Design review of the part built by this model. Coordinates are the model's own, in mm. Coordinates: 2 decimals unless noted, no trailing zeros. Loops run counter-clockwise (first coordinate to the right, second up) from the corner with the lowest first, then second, coordinate; pieces in that order, holes last. Notation, with made-up numbers: (29, 16) - (84, 16) arc R19 ccw to (84, 33) - close; hole circle Ø8 at (89, 75.5). An arc over 180 degrees is marked (long way). One line per question, with ' | ' between items.
from build123d import *

# Parameters (mm, degrees)
SKETCH2_W           = 45.974
SKETCH2_H           = 32.004
BOSS_EXTRUDE1_DEPTH = 21
BOSS_EXTRUDE1_TAPER = 1
CUT_EXTRUDE1_DEPTH  = 36.006658981
SKETCH3_R           = 0.381
BOSS_EXTRUDE2_DEPTH = 8.128


with BuildPart() as part:
    # Sketch2 → Boss-Extrude1 (new body)
    with BuildSketch(Plane.XY):
        Rectangle(SKETCH2_W, SKETCH2_H)
    extrude(amount=BOSS_EXTRUDE1_DEPTH, taper=BOSS_EXTRUDE1_TAPER)

    # Sketch4 → Cut-Extrude1 (cut, through all)
    with BuildSketch(Plane.XY.offset(21)):
        Polygon((-19.177, 16.002), (-22.987, 16.002), (-22.987, 12.192), align=None)
    extrude(amount=-CUT_EXTRUDE1_DEPTH, mode=Mode.SUBTRACT)

    # Sketch3 → Boss-Extrude2 (add)
    with BuildSketch(Plane(origin=(0, 0, 0), x_dir=(-1, 0, 0), z_dir=(0, 0, -1))):
        with Locations(Location((-17.737, 11.998, 0), (0, 0, 180))):
            Circle(SKETCH3_R)
        with Locations(Location((17.763, 3.998, 0), (0, 0, 180))):
            Circle(SKETCH3_R)
        with Locations(Location((17.763, -12.002, 0), (0, 0, 180))):
            Circle(SKETCH3_R)
        with Locations(Location((-17.737, -12.002, 0), (0, 0, 180))):
            Circle(SKETCH3_R)
    extrude(amount=BOSS_EXTRUDE2_DEPTH)


solid = part.part
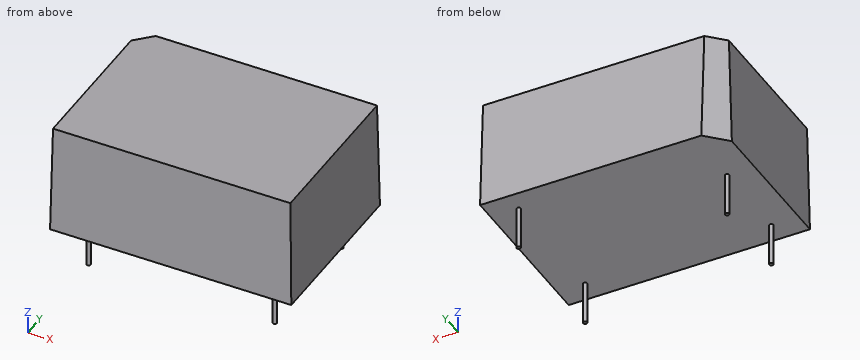
Q1. Take a section at A-A (x = -14). Give the boundary of the cut face in (y, z), plus the area to 3 significant figures.
Returned:
outline: (-16, 0) - (16, 0) - (15.64, 21) - (-15.64, 21) - close | area: 664 mm²
Q2. Take a section at C-C (y = -7). Give the boundary of the cut face in (x, z).
Returned:
outline: (-22.99, 0) - (22.99, 0) - (22.62, 21) - (-22.62, 21) - close
Q3. Take a section at D-D (z = 6). Give the boundary of the cut face in (x, y).
Returned:
outline: (-22.88, -15.9) - (22.88, -15.9) - (22.88, 15.9) - (-19.28, 15.9) - (-22.88, 12.3) - close
Q4. Take a section at B-B (z = 15.5). Give the boundary of the cut face in (x, y).
Returned:
outline: (-22.72, -15.73) - (22.72, -15.73) - (22.72, 15.73) - (-19.45, 15.73) - (-22.72, 12.46) - close
Q5. To check wall thickness, follow line 1 along Z through (x, y) = (-15.5, 11); line 2 along X through (y, z) = (0, 16); line 3 along Y through (x, z) = (2.5, 17). State the ranges of each line that lie inside material, in increasing order.
Returned:
line 1: z = 0 to 21 | line 2: x = -22.71 to 22.71 | line 3: y = -15.71 to 15.71
Q6. For pin 1 (2 mm diameter, centred on x = -9, y = -11, fed in from -Z); pin 2 (1.5 mm diameter, centred on x = 9.5, z = 18, fed in from -Y); pin 3 (1 mm diameter, centred on y = 8.5, z = 11, fed in from +X), all flat-tipped, find the tip position at first contact; note any pin that passes through.
Returned:
pin 1: stops at z = 0 | pin 2: stops at y = -15.7 | pin 3: stops at x = 22.8
